Design review of the part built by this model. Coordinates are the model's own, in mm. Face numbers are marked on the shaded views. A direction names the side the tool comes from. Round coordinates to 2 decimals unless told otherwise and drop trailing zeros. Loops run counter-clockwise (first coordinate to the right, second up) from the corner with the lowest first, then second, coordinate; pieces in that order, holes last. Notation, with made-up numbers: (58, -37) - (74, -37) arc R24 cw to (74, -15) - close; hole circle Ø11 at (71, 14.25). An arc over 180 degrees is marked (long way). Use one line per item in the form item = value. Start each with the question number.
(1) We need section B-B, the plane y = 8. Give the number of separate pieces and of enclosed holes in the cut face, then the cut area to 3 significant figures.
(2) We need section A-A, the plane x = -95. Write out the cut boundary in (y, z).
(3) Machinability: for the marked faces 1 and 2, which of the approach directions +Z, -Z, +X, -X, +Y, -Y give a long, thin tool a straight path to every point of the face, cutting with its end or side? Answer none if there is none.
(4) Wall thickness on probe 1 along Z at (x, y) = (-20.5, 12); probe 2 along Y at (x, z) = (-94, 2); probe 3 along X at (y, z) = (-71.5, 24): over which ranges is each line inside the solid? List them lowest first. Write a range as [from, to].
(5) For pin 1 (14 mm diameter, centred on x = -82, z = 21.5, fed in from -Y); pin 2 (11.5 mm diameter, centred on x = 116.51, y = -199.46, fed in from +Z); pin 3 (0.8 mm diameter, centred on x = -113, z = 1, fed in from +Y), all flat-tipped, find the tip position at first contact; note any pin that passes through.
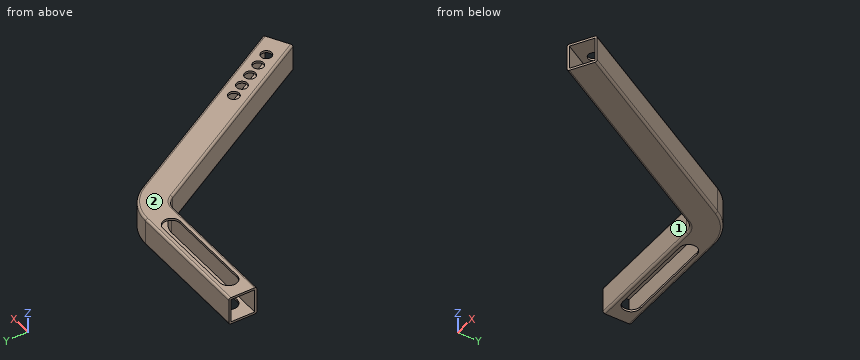
from build123d import *

# Parameters (mm, degrees)
BOSS_EXTRUDE1_DEPTH = 33.02
SHELL1_T            = -2.54
CUT_EXTRUDE1_REACH  = 409.111
SKETCH2_W           = 27.94
SKETCH2_H           = 27.94
CUT_EXTRUDE2_DEPTH  = 2.54
CUT_EXTRUDE3_START  = -2.54
CUT_EXTRUDE3_DEPTH  = 2.54
CUT_EXTRUDE4_REACH  = 303.28
SKETCH5_R           = 6.35
FILLET1_R           = 2.54


with BuildPart() as part:
    # Sketch1 → Boss-Extrude1 (new body)
    with BuildSketch(Plane.XY):
        with BuildLine():
            Line((-172.046968374, 25.4), (-23.576362049, 25.4))
            ThreePointArc((-23.576362049, 25.4), (1.823637951, 18.594090512), (20.417728463, 0))
            Line((20.417728463, 0), (152.4, -228.6))
            Line((152.4, -228.6), (123.803841167, -245.11))
            Line((123.803841167, -245.11), (-8.17843037, -16.51))
            ThreePointArc((-8.17843037, -16.51), (-14.686362049, -10.002068321), (-23.576362049, -7.62))
            Line((-23.576362049, -7.62), (-172.046968374, -7.62))
            Line((-172.046968374, -7.62), (-172.046968374, 25.4))
        make_face()
    extrude(amount=BOSS_EXTRUDE1_DEPTH)

    # Shell1
    shell1_openings = [part.faces().sort_by_distance(p)[0] for p in [
        (-172.046968374, 8.89, 16.51),
    ]]
    offset(amount=SHELL1_T, openings=shell1_openings, kind=Kind.INTERSECTION)

    # Sketch2 → Cut-Extrude1 (cut, up to next)
    with BuildSketch(Plane(origin=(137.086703653, -237.441135768, 0), x_dir=(0.8660254037844406, 0.4999999999999967, 0), z_dir=(0.4999999999999967, -0.8660254037844406, 0)), mode=Mode.PRIVATE) as cut_extrude1_sk1:
        with Locations((1.172271537, 16.51)):
            Rectangle(SKETCH2_W, SKETCH2_H)
    cut_extrude1_tool1 = extrude(cut_extrude1_sk1.sketch, amount=-CUT_EXTRUDE1_REACH, mode=Mode.PRIVATE) & part.part
    add(cut_extrude1_tool1.solids().sort_by_distance((138.101921, -236.855, 16.51))[0], mode=Mode.SUBTRACT)

    # Sketch3 → Cut-Extrude2 (cut)
    with BuildSketch(Plane.XY.offset(33.02)):
        with BuildLine():
            Line((-146.646968374, 19.05), (-45.046968374, 19.05))
            ThreePointArc((-45.046968374, 19.05), (-34.886968374, 8.89), (-45.046968374, -1.27))
            Line((-45.046968374, -1.27), (-50.126968374, -1.27))
            Line((-50.126968374, -1.27), (-146.646968374, -1.27))
            ThreePointArc((-146.646968374, -1.27), (-156.806968374, 8.89), (-146.646968374, 19.05))
        make_face()
    extrude(amount=-CUT_EXTRUDE2_DEPTH, mode=Mode.SUBTRACT)

    # Sketch4 → Cut-Extrude3 (cut)
    with BuildSketch(Plane(origin=(0, 0, 0), x_dir=(-1, 0, 0), z_dir=(0, 0, -1)).offset(CUT_EXTRUDE3_START)):
        with BuildLine():
            Line((141.566968374, -1.27), (146.646968374, -1.27))
            ThreePointArc((146.646968374, -1.27), (156.806968374, 8.89), (146.646968374, 19.05))
            Line((146.646968374, 19.05), (45.046968374, 19.05))
            ThreePointArc((45.046968374, 19.05), (34.886968374, 8.89), (45.046968374, -1.27))
            Line((45.046968374, -1.27), (141.566968374, -1.27))
        make_face()
    extrude(amount=CUT_EXTRUDE3_DEPTH, mode=Mode.SUBTRACT)

    # Sketch5 → Cut-Extrude4 (cut, up to next)
    with BuildSketch(Plane.XY.offset(33.02), mode=Mode.PRIVATE) as cut_extrude4_sk1:
        with Locations((125.401920584, -214.857954744)):
            Circle(SKETCH5_R)
    cut_extrude4_tool1 = extrude(cut_extrude4_sk1.sketch, amount=-CUT_EXTRUDE4_REACH, mode=Mode.PRIVATE) & part.part
    # Sketch5 → Cut-Extrude4 (cut, up to next)
    with BuildSketch(Plane.XY.offset(33.02), mode=Mode.PRIVATE) as cut_extrude4_sk2:
        with Locations((116.511920584, -199.460023065)):
            Circle(SKETCH5_R)
    cut_extrude4_tool2 = extrude(cut_extrude4_sk2.sketch, amount=-CUT_EXTRUDE4_REACH, mode=Mode.PRIVATE) & part.part
    # Sketch5 → Cut-Extrude4 (cut, up to next)
    with BuildSketch(Plane.XY.offset(33.02), mode=Mode.PRIVATE) as cut_extrude4_sk3:
        with Locations((107.621920584, -184.062091385)):
            Circle(SKETCH5_R)
    cut_extrude4_tool3 = extrude(cut_extrude4_sk3.sketch, amount=-CUT_EXTRUDE4_REACH, mode=Mode.PRIVATE) & part.part
    # Sketch5 → Cut-Extrude4 (cut, up to next)
    with BuildSketch(Plane.XY.offset(33.02), mode=Mode.PRIVATE) as cut_extrude4_sk4:
        with Locations((98.731920584, -168.664159706)):
            Circle(SKETCH5_R)
    cut_extrude4_tool4 = extrude(cut_extrude4_sk4.sketch, amount=-CUT_EXTRUDE4_REACH, mode=Mode.PRIVATE) & part.part
    # Sketch5 → Cut-Extrude4 (cut, up to next)
    with BuildSketch(Plane.XY.offset(33.02), mode=Mode.PRIVATE) as cut_extrude4_sk5:
        with Locations((89.841920584, -153.266228027)):
            Circle(SKETCH5_R)
    cut_extrude4_tool5 = extrude(cut_extrude4_sk5.sketch, amount=-CUT_EXTRUDE4_REACH, mode=Mode.PRIVATE) & part.part
    add(cut_extrude4_tool1.solids().sort_by_distance((125.401921, -214.857955, 33.02))[0], mode=Mode.SUBTRACT)
    add(cut_extrude4_tool2.solids().sort_by_distance((116.511921, -199.460023, 33.02))[0], mode=Mode.SUBTRACT)
    add(cut_extrude4_tool3.solids().sort_by_distance((107.621921, -184.062091, 33.02))[0], mode=Mode.SUBTRACT)
    add(cut_extrude4_tool4.solids().sort_by_distance((98.731921, -168.66416, 33.02))[0], mode=Mode.SUBTRACT)
    add(cut_extrude4_tool5.solids().sort_by_distance((89.841921, -153.266228, 33.02))[0], mode=Mode.SUBTRACT)

    # Fillet1
    fillet1_edges = [part.edges().sort_by_distance(p)[0] for p in [
        (57.812705399, -130.81, 0),
        (-14.686362049, -10.002068321, 0),
        (-97.811665212, -7.62, 0),
        (-14.686362049, -10.002068321, 33.02),
        (57.812705399, -130.81, 33.02),
        (86.408864232, -114.3, 33.02),
        (1.823637951, 18.594090512, 33.02),
        (-97.811665212, 25.4, 33.02),
        (-97.811665212, 25.4, 0),
        (-97.811665212, -7.62, 33.02),
        (1.823637951, 18.594090512, 0),
        (86.408864232, -114.3, 0),
    ]]
    fillet(fillet1_edges, radius=FILLET1_R)


solid = part.part
Data:
q1.separate_pieces = 3
q1.enclosed_holes = 0
q1.area = 422 mm^2
q2.outline = (-7.62, 2.54) arc R2.54 ccw to (-5.08, 0) - (-1.27, 0) - (-1.27, 2.54) - (-5.08, 2.54) - (-5.08, 30.48) - (-1.27, 30.48) - (-1.27, 33.02) - (-5.08, 33.02) arc R2.54 ccw to (-7.62, 30.48) - close; (19.05, 0) - (22.86, 0) arc R2.54 ccw to (25.4, 2.54) - (25.4, 30.48) arc R2.54 ccw to (22.86, 33.02) - (19.05, 33.02) - (19.05, 30.48) - (22.86, 30.48) - (22.86, 2.54) - (19.05, 2.54) - close
q3.face_1 = +Z, -Z, -X, -Y
q3.face_2 = +Z, +X, -X, +Y, -Y
q4.probe_1 = [0, 2.54], [30.48, 33.02]
q4.probe_2 = [-7.56, -1.27], [19.05, 25.34]
q4.probe_3 = [23.57, 26.5], [58.77, 61.7]
q5.pin_1 = -7.62
q5.pin_2 = 2.54
q5.pin_3 = 25.13
